Could you check a few things on this model? Use its own coordinates, in mm. A direction names the side the tool comes from. Give positions to 0.01 mm unless a question says otherwise; leave off trailing zeros. Write each loop counter-clockwise with the first axis right and the second up, starting at its lowest first coordinate (ties: lowest second). Pieces come first, ordered by that corner, then holes. Notation, with made-up numbers: M 20,8 L 73,8 A24 cw 73,21 Z; hole C -29.75,7 d1. An arc over 180 degrees is marked long. Write each question's results on one line, items separated by ' | '. Start each with the question number.
from build123d import *

# Parameters (mm, degrees)
BOSS_EXTRUDE1_DEPTH     = 25.4
SKETCH2_R               = 4.7625
CUT_EXTRUDE1_DEPTH      = 1
CUT_EXTRUDE1_DEPTH_BACK = 26.4


with BuildPart() as part:
    # Sketch1 → Boss-Extrude1 (new body)
    with BuildSketch(Plane(origin=(0, 0, 0), x_dir=(1, 0, 0), z_dir=(0, 1, 0))):
        Polygon((101.6, 0), (-101.6, 0), (-101.6, 50.8), (-76.2, 76.2), (-76.2, 25.4), (76.2, 25.4), (76.2, 76.2), (101.6, 50.8), align=None)
        Polygon((-76.2, 76.2), (-61.959231637, 90.440768363), (-79.919743879, 108.401280605), (-133.801280605, 54.519743879), (-115.840768363, 36.559231637), (-101.6, 50.8), align=None)
        Polygon((101.6, 50.8), (76.2, 76.2), (61.959231637, 90.440768363), (79.919743879, 108.401280605), (133.801280605, 54.519743879), (115.840768363, 36.559231637), align=None)
    extrude(amount=BOSS_EXTRUDE1_DEPTH)

    # Sketch2 → Cut-Extrude1 (cut, two sides)
    with BuildSketch(Plane(origin=(0, 25.4, 0), x_dir=(1, 0, 0), z_dir=(0, 1, 0))) as cut_extrude1_sk:
        with Locations((25.4, 12.7)):
            Circle(SKETCH2_R)
        with Locations((-25.4, 12.7)):
            Circle(SKETCH2_R)
    extrude(amount=CUT_EXTRUDE1_DEPTH, mode=Mode.SUBTRACT)
    extrude(cut_extrude1_sk.sketch, amount=-CUT_EXTRUDE1_DEPTH_BACK, mode=Mode.SUBTRACT)


solid = part.part
Q1. I'm going to push flat-ended pins straight in: P1, Ø11, axis at x = -25.4, z = -12.7, coming from the +Y side; P2, Ø8, axis at y = 15.5, z = -87.5, coming from the +X side; P3, Ø2, axis at x = 51.5, y = 5, coming from the -Z side; P4, Ø12.5, axis at y = 13, z = -38.5, coming from the +X side. Where does each tip first touch, or does it pass through?
Q2. If we section it at A-A (x = 25.4): Please give me the cut outline in (y, z), plus the area to 3 significant figures.
Q3. If we section it at D-D (z = -33): Please give me the cut outline in (x, y), plus the area to 3 significant figures.
Q4. If we section it at B-B (z = -12.7): Please give me the cut outline in (x, y).
Q5. For faces 1 (the face through (101.6, 13, -26)), 2 (the face through (70.814, 12.522, -99.295)), 3 (the face through (-76.2, 13, -51)), which set-ups out of +Z, -Z, +X, -X, +Y, -Y let a thin tool reach every point of the face, with its end or its side?
Q6. If we section it at C-C (y = 15.25): Please give me the cut outline in (x, z) (1 decimal).
Q7. If we mould it in two halves opening along Z, with no side actions, what happens to faces 4 (the face through (1, 13, 0)), 5 (the face through (76.2, 13, -50)), 6 (the face through (-106.48, 12.52, -81.84))? For each: pulls with the +Z half, pulls with the -Z half, needs draft (parallel to the pull), parting line crosses it, or undercut.
Q8. Please list where these lines run through material, in increasing order: line 1 (X direction, y = 13.5, z = -12.7); line 2 (Z direction, x = -25.4, y = 10.25); line 3 (X direction, y = 15.25, z = -39). Write a range as [from, to].
Determined:
1) P1: stops at y = 25.4 | P2: stops at x = 104.82 | P3: stops at z = -25.4 | P4: stops at x = 124.03
2) outline: M 0,-25.4 L 25.4,-25.4 L 25.4,-17.46 L 0,-17.46 Z; M 0,-7.94 L 25.4,-7.94 L 25.4,0 L 0,0 Z | area: 403 mm²
3) outline: M -101.6,0 L -76.2,0 L -76.2,25.4 L -101.6,25.4 Z; M 76.2,0 L 101.6,0 L 101.6,25.4 L 76.2,25.4 Z | area: 1,290 mm²
4) outline: M -101.6,0 L -30.16,0 L -30.16,25.4 L -101.6,25.4 Z; M -20.64,0 L 20.64,0 L 20.64,25.4 L -20.64,25.4 Z; M 30.16,0 L 101.6,0 L 101.6,25.4 L 30.16,25.4 Z
5) face 1: +Z, +Y, -Y | face 2: -Z, +Y, -Y | face 3: +Y, -Y
6) outline: M -133.8,-54.5 L -79.9,-108.4 L -62,-90.4 L -76.2,-76.2 L -76.2,-25.4 L 76.2,-25.4 L 76.2,-76.2 L 62,-90.4 L 79.9,-108.4 L 133.8,-54.5 L 115.8,-36.6 L 101.6,-50.8 L 101.6,0 L -101.6,0 L -101.6,-50.8 L -115.8,-36.6 Z; hole C -25.4,-12.7 d9.5; hole C 25.4,-12.7 d9.5
7) face 4: pulls with the +Z half | face 5: undercut | face 6: pulls with the -Z half
8) line 1: x = [-101.6, -30.16], [-20.64, 20.64], [30.16, 101.6] | line 2: z = [-25.4, -17.46], [-7.94, 0] | line 3: x = [-118.28, -113.4], [-101.6, -76.2], [76.2, 101.6], [113.4, 118.28]
